Input: part model. Units: mm. Frame: model coordinates. Face numbers are marked on the shaded views. A direction names the side the tool comes from. Round coordinates to 2 decimals unless told otherwise and drop trailing zeros. Write each loop counter-clockwise with the first axis right and the second up, starting at its lowest first coordinate (ties: lowest second). Pieces come first, ordered by that corner, then holes. Notation, with made-up numbers: (47, 29) -> (61, 29) arc R19 ccw to (61, 41) -> close; hole circle Ø1 at (2.5, -16). An arc over 180 degrees is marked (long way). Write item = value, one per line.
Autodesk Inventor part; units mm, degrees
ref_plane "YZ Plane" through (0, 0, 0) normal (1, 0, 0) x (0, 1, 0)
ref_plane "XZ Plane" through (0, 0, 0) normal (0, 1, 0) x (-1, 0, 0)
ref_plane "XY Plane" through (0, 0, 0) normal (0, 0, 1) x (1, 0, 0)
sketch "Sketch1" plane through (0, 0, 0) normal (0, 0, 1) x (1, 0, 0)
  line L0 (-12.2264, 9.7457) -> (-5.1779, 13.8152)
  line L1 (-5.1779, 13.8152) -> (1.8706, 9.7457)
  line L2 (1.8706, 9.7457) -> (1.8706, 1.6068)
  line L3 (1.8706, 1.6068) -> (-5.1779, -2.4626)
  line L4 (-5.1779, -2.4626) -> (-12.2264, 1.6068)
  line L5 (-12.2264, 1.6068) -> (-12.2264, 9.7457)
  point P0 (0, 0)
  point P1 (-5.1779, 5.6763)
  dimension "d0" = 14.097
extrude "Extrusion1" add sketch "Sketch1" along normal blind 8.255
sketch "Sketch2" plane through (0, 0, 8.255) normal (0, 0, 1) x (1, 0, 0)
  circle A0 centre (-5.1779, 5.6763) radius 6.8961
  point P0 (0, 0)
  dimension "d3" = 13.7922
extrude "Extrusion2" add sketch "Sketch2" along normal blind 3.048
sketch "Sketch3" plane through (-5.1779, 5.6763, 11.303) normal (0, 0, 1) x (1, 0, 0)
  circle A0 centre (0, 0) radius 6.8961
  circle A1 centre (0, 0) radius 4.0005
  point P0 (5.1779, -5.6763)
  dimension "d6" = 8.001
extrude "Extrusion3" cut sketch "Sketch3" against normal through all contours A1
thread "Thread1"
properties part number "Big Nut 1764"
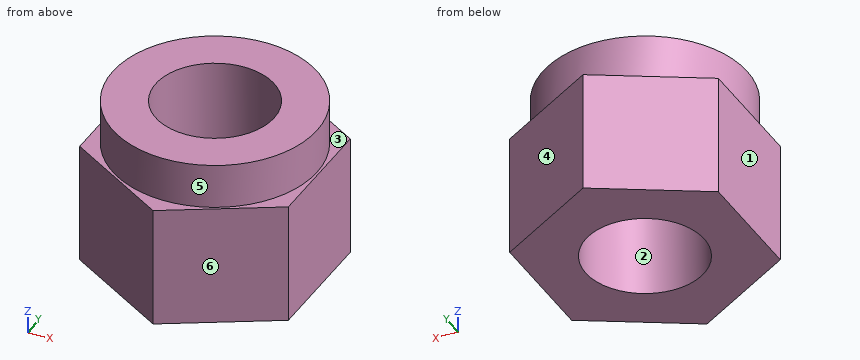
1) First-contact query: P1, Ø5, axis at x = -7, z = 4.5, coming from the -Y side; P2, Ø1.5, axis at y = 7.5, z = 9.5, coming from the +X side; P3, Ø1, axis at x = -6.5, z = 9.5, coming from the -Y side. Flat tips, straight axial feed; report the tip coordinate or a pass-through.
Solutions:
P1 = -2.46
P2 = 1.63
P3 = -1.17
2) Draft query along X for the marked faces 1, 2, 3 and 4. Return one class per face: +X half, -X half, draft (parallel to the pull), parting line (faces both ways), or undercut.
Solutions:
face_1 = -X half
face_2 = undercut
face_3 = draft
face_4 = +X half
3) Cut plane B-B (z = 3.25). Return the cut outline in (x, y), and give its area (3 significant figures).
Solutions:
outline = (-12.23, 1.61) -> (-5.18, -2.46) -> (1.87, 1.61) -> (1.87, 9.75) -> (-5.18, 13.82) -> (-12.23, 9.75) -> close; hole circle Ø8 at (-5.18, 5.68)
area = 122 mm^2
4) Line query: L1, parallel to X at y = 4.5, z = 8; L2, parallel to X at y = 5.25, z = 7; L3, parallel to Y at x = -7, z = 9.75. Output: solid intervals per line, ascending. Write a range as from..to.
Solutions:
L1 = -12.23..-9, -1.35..1.87
L2 = -12.23..-9.16, -1.2..1.87
L3 = -0.97..2.11, 9.24..12.33
5) Cut plane D-D (x = 0). Return the cut outline in (y, z) (3 decimals).
Solutions:
outline = (0.527, 0) -> (10.826, 0) -> (10.826, 8.255) -> (10.231, 8.255) -> (10.231, 11.303) -> (1.122, 11.303) -> (1.122, 8.255) -> (0.527, 8.255) -> close
6) Cut plane A-A (x = -1.75). Return the cut outline in (y, z) (3 decimals), and give its area (3 significant figures).
Solutions:
outline = (-0.484, 0) -> (3.614, 0) -> (3.614, 11.303) -> (-0.307, 11.303) -> (-0.307, 8.255) -> (-0.484, 8.255) -> close; (7.739, 0) -> (11.836, 0) -> (11.836, 8.255) -> (11.66, 8.255) -> (11.66, 11.303) -> (7.739, 11.303) -> close
area = 91.6 mm^2
7) Cut plane C-C (y = 6.5). Return the cut outline in (x, z) (3 decimals).
Solutions:
outline = (-12.226, 0) -> (-9.093, 0) -> (-9.093, 11.303) -> (-12.025, 11.303) -> (-12.025, 8.255) -> (-12.226, 8.255) -> close; (-1.263, 0) -> (1.871, 0) -> (1.871, 8.255) -> (1.669, 8.255) -> (1.669, 11.303) -> (-1.263, 11.303) -> close
8) Access query for the marked faces 5 and 6. Directions: +Z, -Z, +X, -X, +Y, -Y. A direction counts if a zero-diameter tool reaches every point of the face in a straight line with its end or side. Return the directions, or none.
Solutions:
face_5 = +Z
face_6 = +Z, -Z, +X, -Y
